Could you check a few things on this model? Use its own coordinates, in mm. A direction names the side the tool comes from. Give positions to 0.01 mm unless a question says otherwise; leave off trailing zeros. Order: outer loops, then holes, each group sorted by start corner. A loop starts at its lowest first (then second) coordinate and runs counter-clockwise, first axis right, second up. Notation, with made-up numbers: M 29,73.25 L 42,73.25 A19 cw 42,106.25 Z; hole C -22.75,-23.75 d7. An arc over 180 degrees is marked long. Answer in a Markdown table with one row per item. Add a question column.
Autodesk Inventor part; units mm, degrees
ref_plane "YZ Plane" through (0, 0, 0) normal (1, 0, 0) x (0, 1, 0)
ref_plane "XZ Plane" through (0, 0, 0) normal (0, 1, 0) x (-1, 0, 0)
ref_plane "XY Plane" through (0, 0, 0) normal (0, 0, 1) x (1, 0, 0)
sketch "Sketch1" plane through (0, 0, 0) normal (0, 1, 0) x (-1, 0, 0)
  circle A0 centre (0, 0) radius 1.5
  circle A1 centre (0, 0) radius 8.5
  dimension "d0" = 3
  dimension "d1" = 17
extrude "Extrusion1" add sketch "Sketch1" along normal blind 8
chamfer "Chamfer1" distance 0.5 distance2 7 1 edges at (1.5, 8, 0) measured on face at (-6.0698, 8, -0.7977)
sketch "Sketch2" plane through (0, 0, 0) normal (0, -1, 0) x (1, 0, 0)
  circle A0 centre (0, 0) radius 8.5
extrude "Extrusion2" add sketch "Sketch2" along normal blind 1
fillet "Fillet1" radius 2 1 edges at (-8.5, -1, 0)
sketch "Sketch3" plane through (0, 8, 0) normal (0, 1, 0) x (1, 0, 0)
  circle A0 centre (0, 0) radius 2
  circle A1 centre (0, 0) radius 3.5
  dimension "d10" = 7
extrude "Extrusion3" cut sketch "Sketch3" against normal blind 1 contours A0 | A1
sketch "Sketch4" plane through (0, 7, 0) normal (0, 1, 0) x (1, 0, 0)
  circle A0 centre (0, 0) radius 1.9286
  circle A1 centre (0, 0) radius 3.5
  circle A2 centre (0, 0) radius 2
  dimension "d13" = 4
extrude "Extrusion4" add sketch "Sketch4" along normal blind 1 contours A2
chamfer "Chamfer2" distance 0.5 angle 45 1 edges at (-3.5, 7, 0)
equation "\"BendRadius\" = Thickness"
equation "\"BendReliefWidth\" = Thickness"
equation "\"BendReliefDepth\" = 0.5 * Thickness"
equation "\"CornerReliefSize\" = 4 * Thickness"
equation "\"MinimumRemnant\" = 2 * Thickness"
equation "\"TransitionRadius\" = BendRadius"
equation "\"JacobiRadiusSize\" = BendRadius"
equation "\"GapSize\" = Thickness"
properties part number "powerButtonPart1"
1. Thinking about a two-plate mould opening in Z: for faces 3 (the flat face through (0, -1, 0)), 4 (the cylindrical face through (-4.57, 4.451, -7.167)), 5 (the flat face through (1, 7, 2)), which applies, pulls with the +Z half, pulls with the -Z half, needs draft (parallel to the pull), parting line crosses it, or undercut?
2. If I drill on line 1 along X through (y, z) = (1.25, -0.25); line 2 along X through (y, z) = (0.25, -0.25); line 3 along Y through (x, z) = (2.5, 1), over which ranges is the centre line in solid material (lowest first)? Write a range as [from, to].
3. Will this pin go through, and if not, where does the flat tip stop? P1, Ø2.5, axis at x = 0, z = 0, coming from the +Y side.
4. Suppose I cut it at A-A on y = 3. List the corners of the cut face in (x, z) for me, plus the area to 3 significant figures.
5. For faces 1 (the flat face through (-4, 8, 0)), 2 (the flat face through (0, 0, 0)), which set-ups out of +Z, -Z, +X, -X, +Y, -Y let a thin tool reach every point of the face, with its end or its side?
6. Suppose I cut it at B-B on y = 5. List the corners of the cut face in (x, z) for me.
Findings below:
| question | item | result |
|---|---|---|
| 1 | face 3 | needs draft |
| 1 | face 4 | parting line crosses it |
| 1 | face 5 | undercut |
| 2 | line 1 | [-8.5, -1.5], [1.5, 8.5] |
| 2 | line 2 | [-8.35, -1.48], [1.48, 8.35] |
| 2 | line 3 | [-1, 7] |
| 3 | P1 | y = 0 |
| 4 | outline | C 0,0 d17; hole C 0,0 d3.29 |
| 4 | area | 219 mm2 |
| 5 | face 1 | +Z, -Z, +X, -X, +Y |
| 5 | face 2 | +Y |
| 6 | outline | C 0,0 d17; hole C 0,0 d3.57 |
